Here's the drawing with two shaded views (mm, measured from the low corner). I have some questions. A direction names the side the tool comes from. Round coordinates to 2 decimals unless told otherwise and drop trailing zeros. Loops run counter-clockwise (first coordinate to the right, second up) from the corner with the lowest first, then second, coordinate; pieces in that order, holes last. Notation, with made-up numbers: (36.25, 87) - (88.25, 87) arc R17 ccw to (88.25, 98) - close; hole circle Ø7 at (-4.75, -33). An arc over 180 degrees is marked (long way). Use one line per item in the form item = value.
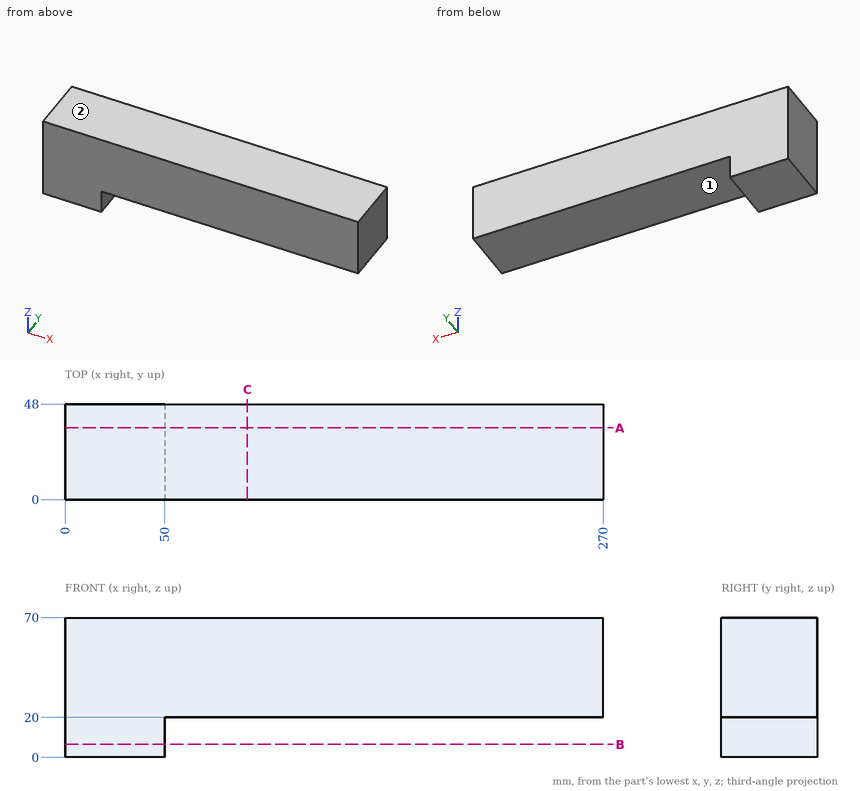
1. If we section it at C-C, the plane x = 91.5: Write out the boundary of the cut face in (y, z), plus the area to 3 significant figures.
Solution:
outline = (0, 20) - (48, 20) - (48, 70) - (0, 70) - close
area = 2,400 mm^2
2. If we section it at B-B, the plane z = 6.5: Write out the boundary of the cut face in (x, y), plus the area to 3 significant figures.
Solution:
outline = (0, 0) - (50, 0) - (50, 48) - (0, 48) - close
area = 2,400 mm^2
3. For P1, Ø6, axis at y = 15.5, z = 9, coming from the +X side, with a flat end and sliding along its axis, tell me the tip position at first contact or that it passes through.
Solution:
P1 = 50
4. On a 3-axis mill with a long thin cutter (end or side, diameter ignored), from which of +Z, -Z, +X, -X, +Y, -Y can I reach the whole of each face in a straight line? I mean the marked faces 1 and 2. Say none if no direction works.
Solution:
face_1 = -Z, +X, +Y, -Y
face_2 = +Z, +X, -X, +Y, -Y
5. Please list where these lines run through material, in increasing order: line 1 along Z through (x, y) = (150, 30); line 2 along X through (y, z) = (40.5, 6.5).
Solution:
line_1 = 20 to 70
line_2 = 0 to 50
6. If we section it at A-A, the plane y = 36: Write out the boundary of the cut face in (x, z).
Solution:
outline = (0, 0) - (50, 0) - (50, 20) - (270, 20) - (270, 70) - (0, 70) - close
